Here's the drawing with two shaded views (mm, measured from the low corner). I have some questions. Give positions to 0.01 mm unless a question says otherwise; leave off trailing zeros. Loops run counter-clockwise (first coordinate to the right, second up) from the corner with the lowest first, then second, coordinate; pieces in that order, holes last. Notation, with made-up numbers: M 49,-4.5 L 55,-4.5 A16 ccw 55,5.5 Z; hole C 15,-0.5 d10. An arc over 180 degrees is marked long. Put each result on its own line as item: value. Start each with the question number.
1) Imagine slicing it at D-D (z = 14.25). Write out the boundary of the cut face in (x, y) (1 decimal).
2) Imagine slicing it at C-C (y = 0.2). Write out the boundary of the cut face in (x, z) (1 decimal).
3) For P1, Ø0.8, axis at x = 9, y = 0.5, coming from the -Z side; P2, Ø0.5, axis at x = 11.5, y = 0.5, coming from the +Z side, each with a flat end and sliding along its axis, tell me the tip position at first contact or that it passes through.
4) Imagine slicing it at B-B (z = 8). Write out the boundary of the cut face in (x, y) (1 decimal).
5) Please list where these lines run through material, in increasing order: line 1 along X through (y, z) = (0.8, 9.5); line 2 along Z through (x, y) = (8, 0.85); line 3 along Z through (x, y) = (3.25, 0.1) (1 decimal). Write a range as from..to.
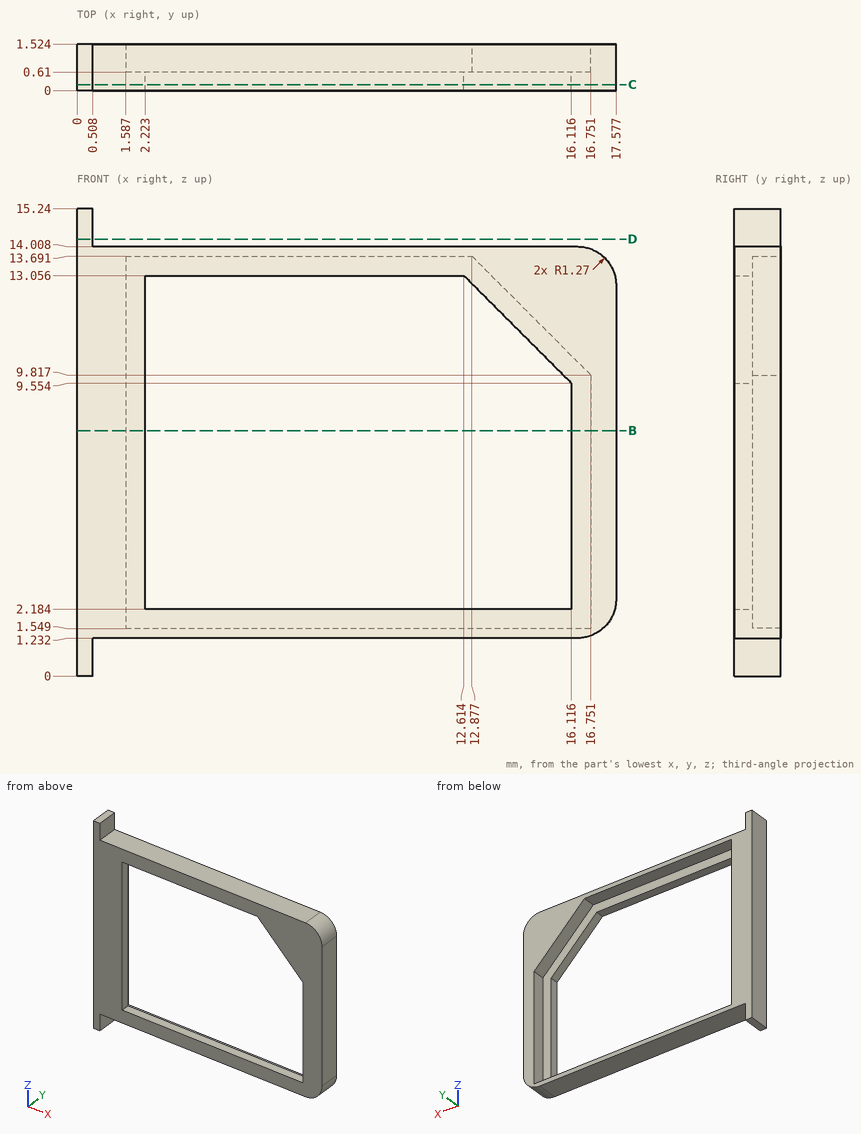
Recorded:
1. outline: M 0,0 L 0.5,0 L 0.5,1.5 L 0,1.5 Z
2. outline: M 0,0 L 0.5,0 L 0.5,1.2 L 16.3,1.2 A1.3 ccw 17.6,2.5 L 17.6,12.7 A1.3 ccw 16.3,14 L 0.5,14 L 0.5,15.2 L 0,15.2 Z; hole M 2.2,2.2 L 16.1,2.2 L 16.1,9.6 L 12.6,13.1 L 2.2,13.1 Z
3. P1: z = 1.23
3. P2: z = 14.01
4. outline: M 0,0 L 2.2,0 L 2.2,0.6 L 1.6,0.6 L 1.6,1.5 L 0,1.5 Z; M 16.1,0 L 17.6,0 L 17.6,1.5 L 16.8,1.5 L 16.8,0.6 L 16.1,0.6 Z
5. line 1: 0..1.59, 16.75..17.58
5. line 2: 1.23..1.55, 13.69..14.01
5. line 3: 1.2..2.2, 13.1..14
